Autodesk Inventor part; units mm, degrees
sketch "スケッチ1" plane through (0, 0, 0) normal (0, 0, 1) x (1, 0, 0)
  circle A0 centre (0, 0) radius 140
  arc A1 (-6.6994, 21.4795) -> (7, 21.3834) centre (0, 0) ccw
  line L0 (0, 22.5) -> (0, 17)
  line L1 (0, 22.5) -> (0, 26.3)
  line L2 (0, 26.3) -> (7, 26.3)
  line L3 (7, 26.3) -> (7, 21.3834)
  line L4 (7, 17) -> (0, 17)
  line L5 (-6.6994, 21.4795) -> (-6.6994, 26.3)
  line L6 (-6.6994, 26.3) -> (0, 26.3)
  dimension "d0" = 280
  dimension "d1" = 45
  dimension "d2" = 5.5
  dimension "d3" = 3.8
  dimension "d4" = 7
extrude "押し出し1" add sketch "スケッチ1" along normal blind 40
properties part number "gear2"
Build history of the part. All positions in model axes, mm. Coordinates: 2 decimals unless noted, no trailing zeros. Order: outer loops, then holes, each group sorted by start corner. A loop starts at its lowest first (then second) coordinate and runs counter-clockwise, first axis right, second up. Notation, with made-up numbers: M -14,19 L 37,19 A23 cw 37,35 Z; hole C 64,-16 d7. An arc over 180 degrees is marked long. One line per question, with ' | ' between items. Start each with the question number.
Q1. Probe L1, parallel to Y at x = -7, z = 12.5; L2, parallel to X at y = -19.5, z = 5; L3, parallel to X at y = 119.5, z = 28.5. List the from-to ranges inside material, lowest first. Write a range as from..to.
Q2. Two-plate mould, pull along X, no slides. Class faces 1 (the face through (0, 26.3, 20)), 2 (the face through (-2, -29, 40)), 3 (the face through (-111.1, 85.19, 19.72)), 4 (the face through (0.73, -22.49, 19.72)): +X half, -X half, draft (parallel to the pull), parting line (faces both ways), or undercut.
Q3. Saw through at B-B (y = 0). List the corners of the cut face in (x, z), then the cut area to 3 significant figures.
Q4. Saw through at C-C (z = 29). List the corners of the cut face in (x, y), then the cut area to 3 significant figures.
Q5. Saw through at D-D (y = 41.5). List the corners of the cut face in (x, z), then the cut area to 3 significant figures.
Q6. Flat gauge pins, fed straight in: pin 1 Ø4 at (x, z) = (23, 20) entering from -Y; pin 2 Ø4 at (y, z) = (23.5, 27.5) entering from +X; pin 3 Ø1.5 at (x, z) = (16, 26) entering from -Y. Where does each tip first touch, or does it go through?
Q7. Saw through at A-A (x = 0). List the corners of the cut face in (y, z), then the cut area to 3 significant figures.
Check values:
1) L1: y = -139.82..-21.38, 21.38..139.82 | L2: x = -138.64..-11.23, 11.22..138.64 | L3: x = -72.94..72.94
2) face 1: undercut | face 2: draft | face 3: parting line | face 4: undercut
3) outline: M -140,0 L -22.5,0 L -22.5,40 L -140,40 Z; M 22.5,0 L 140,0 L 140,40 L 22.5,40 Z | area: 9,400 mm2
4) outline: C 0,0 d280; hole M -6.7,21.48 A22.5 ccw long 7,21.38 L 7,26.3 L -6.7,26.3 Z | area: 59,900 mm2
5) outline: M -133.71,0 L 133.71,0 L 133.71,40 L -133.71,40 Z | area: 10,700 mm2
6) pin 1: stops at y = -138.42 | pin 2: stops at x = 138.34 | pin 3: stops at y = -139.17
7) outline: M -140,0 L -22.5,0 L -22.5,40 L -140,40 Z; M 26.3,0 L 140,0 L 140,40 L 26.3,40 Z | area: 9,250 mm2
